Solid Edge part; units mm, degrees
sketch "Sketch1" plane through (0, 0, 0) normal (0, 0, 1) x (1, 0, 0)
  line L0 (30, -49.2434) -> (-30, -49.2434)
  line L1 (-30, -49.2434) -> (-30, 40.7566)
  line L2 (-30, 40.7566) -> (30, 40.7566)
  line L3 (30, 40.7566) -> (30, -49.2434)
  dimension "D1" = 30
  dimension "D2" = 30
extrude "Protrusion1" add sketch "Sketch1" along normal blind 7
chamfer "Chamfer_1" distance 4.6 angle 45 4 edges at (0, -49.2434, 7) (30, -4.2434, 7) (0, 40.7566, 7) (-30, -4.2434, 7)
fillet "Round_1" radius 3 8 edges at (-27.7, 38.4566, 4.7) (0, 36.1566, 7) (-25.4, -4.2434, 7) (-27.7, -46.9434, 4.7) (0, -44.6434, 7) (27.7, -46.9434, 4.7) (25.4, -4.2434, 7) (27.7, 38.4566, 4.7)
shell "Thinwall_1" thickness 1.5 removed faces 1 at (20.6, -33.3434, 0)
sketch "Sketch2" plane through (0, -4.1731, 5.5) normal (0, 0, -1) x (-1, 0, 0)
  circle A0 centre (-12.3176, 26.7231) radius 1
  circle A1 centre (12.1907, 26.7231) radius 1
  circle A2 centre (16.82, -10.0727) radius 1
  circle A3 centre (-16.82, -10.0727) radius 1
extrude "ExtrudedProtrusion_2" add sketch "Sketch2" along normal blind 4
sketch "Sketch3" plane through (0, 0, 0) normal (0, 0, 1) x (1, 0, 0)
  line L0 (-23, 29.6566) -> (-30, 29.6566)
  line L1 (-30, 29.6566) -> (-30, 40.7566)
  line L2 (-18.9, 40.7566) -> (-30, 40.7566)
  line L3 (-18.9, 33.7566) -> (-18.9, 40.7566)
  arc A0 (-23, 29.6566) -> (-18.9, 33.7566) centre (-23, 33.7566) ccw
  line L4 (18.9, 33.7566) -> (18.9, 40.7566)
  line L5 (18.9, 40.7566) -> (30, 40.7566)
  line L6 (30, 29.6566) -> (30, 40.7566)
  line L7 (23, 29.6566) -> (30, 29.6566)
  arc A1 (18.9, 33.7566) -> (23, 29.6566) centre (23, 33.7566) ccw
  line L8 (23, -38.1434) -> (30, -38.1434)
  line L9 (30, -38.1434) -> (30, -49.2434)
  line L10 (18.9, -49.2434) -> (30, -49.2434)
  line L11 (18.9, -42.2434) -> (18.9, -49.2434)
  arc A2 (23, -38.1434) -> (18.9, -42.2434) centre (23, -42.2434) ccw
  line L12 (-23, -38.1434) -> (-30, -38.1434)
  line L13 (-30, -38.1434) -> (-30, -49.2434)
  line L14 (-18.9, -49.2434) -> (-30, -49.2434)
  line L15 (-18.9, -42.2434) -> (-18.9, -49.2434)
  arc A3 (-23, -38.1434) -> (-18.9, -42.2434) centre (-23, -42.2434) cw
  dimension "D1" = 23
  dimension "D2" = 23
  dimension "D3" = 23
  dimension "D4" = 23
extrude "Protrusion2" add sketch "Sketch3" along normal up to next
sketch "Sketch4" plane through (0, -4.4902, 1) normal (0, 0, -1) x (-1, 0, 0)
  circle A0 centre (-23, -37.7532) radius 4.1
  circle A1 centre (23, -37.7532) radius 4.1
  circle A2 centre (23, 38.2468) radius 4.1
  circle A3 centre (-23, 38.2468) radius 4.1
extrude "ExtrudedCutout_1" cut sketch "Sketch4" against normal blind 3
sketch "Sketch5" plane through (0, -4.2434, 0) normal (0, 0, -1) x (-1, 0, 0)
  circle A0 centre (-23, -38) radius 1.5
  circle A1 centre (23, -38) radius 1.5
  circle A2 centre (23, 38) radius 1.5
  circle A3 centre (-23, 38) radius 1.5
extrude "ExtrudedCutout_2" cut sketch "Sketch5" against normal blind 5
sketch "Sketch6" plane through (0, -49.2434, 1.2) normal (0, -1, 0) x (-1, 0, 0)
  line L0 (-3.34, -0.8) -> (4.66, -0.8)
  line L1 (5.66, 0.2) -> (5.66, 1.2)
  line L2 (5.66, 1.2) -> (-4.34, 1.2)
  line L3 (-4.34, 0.2) -> (-4.34, 1.2)
  arc A0 (4.66, -0.8) -> (5.66, 0.2) centre (4.66, 0.2) ccw
  arc A1 (-4.34, 0.2) -> (-3.34, -0.8) centre (-3.34, 0.2) ccw
  dimension "D1" = 3.34
extrude "Cutout1" cut sketch "Sketch6" against normal up to next
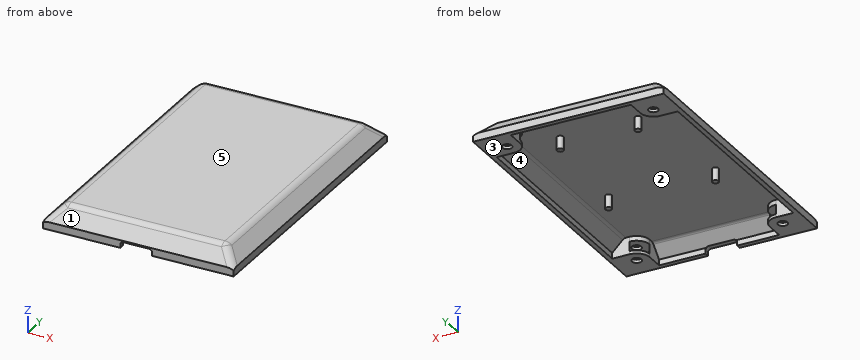
The listing builds one solid part. Answer for the finished solid, in the listing's coordinates (mm). Face numbers are marked on the shaded views. A direction names the side the tool comes from. Coordinates: 2 decimals unless noted, no trailing zeros. Write each loop counter-clockwise with the first axis right and the second up, starting at its lowest first coordinate (ties: lowest second). Pieces come first, ordered by that corner, then holes. Notation, with made-up numbers: (72, 50) - (83, 50) arc R24 cw to (83, 77) - close; hole circle Ø3 at (60, -30). An arc over 180 degrees is marked (long way). Return JSON: item names as keys, results as strings. Group by question number.
Q1. The part is cut by section B-B on x = -16.82. Write down the section's boundary in (y, z), and give its area (3 significant figures).
Q2. For a pull along Y with two mould halves and no side action, classify the marked faces 1, 2 and 3 as +Y half, -Y half, draft (parallel to the pull), parting line (faces both ways), or undercut.
Q3. The part is cut by section A-A on y = 22.55. Write down the section's boundary in (x, z), and give its area (3 significant figures).
Q4. Flat-ended cylindrical pins translate along their axes: pin 1 Ø3 at (y, z) = (-35.5, 5) entering from -X; pin 2 Ø4 at (y, z) = (-12.5, 2.5) entering from +X; pin 3 Ø3 at (x, z) = (-25.5, 4) entering from +Y; pin 4 Ø5 at (x, y) = (16, 11.5) entering from -Z. Find the tip coordinate at first contact, or state that the pin passes through.
Q5. Find the intervals of material crossed by line 1 along Y through (x, z) = (23, 4.5); line 2 along Y through (x, z) = (-23, 4.3); line 3 along Y through (x, z) = (13, 3), in increasing order. Write a range as [from, to].
Q6. Which of the six approach directions +Z, -Z, +X, -X, +Y, -Y give full straight-line access (tool end or side, diameter ignored) to the marked faces 4 and 5?
Q7. The part is cut by section C-C on y = -18.5. Write down the section's boundary in (x, z), and give its area (3 significant figures).
Evaluation:
{
 "1": {"outline": "(-49.24, 0) - (-47.74, 0) - (-47.74, 1.78) - (-44.46, 5.06) arc R1.5 cw to (-43.4, 5.5) - (-15.25, 5.5) - (-15.25, 1.5) - (-13.25, 1.5) - (-13.25, 5.5) - (34.91, 5.5) arc R1.5 cw to (35.97, 5.06) - (39.26, 1.78) - (39.26, 0) - (40.76, 0) - (40.76, 2.4) - (37.04, 6.12) arc R3 ccw to (34.91, 7) - (-43.4, 7) arc R3 ccw to (-45.52, 6.12) - (-49.24, 2.4) - close", "area": "152 mm2"},
 "2": {"face 1": "-Y half", "face 2": "undercut", "face 3": "draft"},
 "3": {"outline": "(-30, 0) - (-28.5, 0) - (-28.5, 1.78) - (-25.22, 5.06) arc R1.5 cw to (-24.16, 5.5) - (-13.19, 5.5) - (-13.19, 1.5) - (-11.19, 1.5) - (-11.19, 5.5) - (11.32, 5.5) - (11.32, 1.5) - (13.32, 1.5) - (13.32, 5.5) - (24.16, 5.5) arc R1.5 cw to (25.22, 5.06) - (28.5, 1.78) - (28.5, 0) - (30, 0) - (30, 2.4) - (26.28, 6.12) arc R3 ccw to (24.16, 7) - (-24.16, 7) arc R3 ccw to (-26.28, 6.12) - (-30, 2.4) - close", "area": "115 mm2"},
 "4": {"pin 1": "stops at x = -28.9", "pin 2": "stops at x = 30", "pin 3": "stops at y = 40.66", "pin 4": "stops at z = 5.5"},
 "5": {"line 1": "y = [-47.14, -43.74], [-40.74, -38.14], [29.66, 32.26], [35.26, 38.66]", "line 2": "y = [-47.34, -43.74], [-40.74, -38.14], [29.66, 32.26], [35.26, 38.86]", "line 3": "y = [-48.64, -46.52], [21.82, 23.28], [38.04, 40.16]"},
 "6": {"face 4": "-Z", "face 5": "+Z, +X, -X, +Y, -Y"},
 "7": {"outline": "(-30, 0) - (-28.5, 0) - (-28.5, 1.78) - (-25.22, 5.06) arc R1.5 cw to (-24.16, 5.5) - (24.16, 5.5) arc R1.5 cw to (25.22, 5.06) - (28.5, 1.78) - (28.5, 0) - (30, 0) - (30, 2.4) - (26.28, 6.12) arc R3 ccw to (24.16, 7) - (-24.16, 7) arc R3 ccw to (-26.28, 6.12) - (-30, 2.4) - close", "area": "98.9 mm2"}
}
